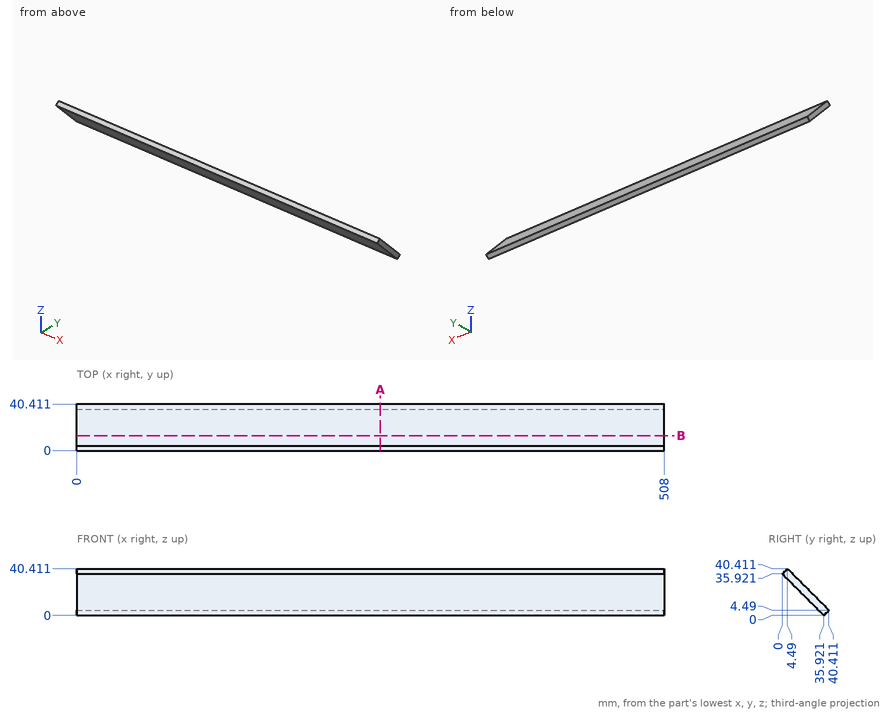
Verification items for this drawing (mm, ordinates from the low corner). Give positions to 0.01 mm unless a question says otherwise; leave off trailing zeros. Write each loop counter-clockwise with the first axis right and the second up, starting at its lowest first coordinate (ties: lowest second). Pieces come first, ordered by that corner, then holes.
1) Section check A-A, the plane x = 262.5. Record the boundary of the cut face in (y, z), and give its area (3 significant figures).
2) Material ranges on L1, parallel to Y at x = 208, z = 8.5; L2, parallel to Y at x = 54, z = 37; L3, parallel to Z at x = 226, y = 27, recorded low to high.
3) Gauge pin test, flat ends, axial feed: pin 1 (1 mm diameter, centred on x = 182.5, z = 27.5, fed in from +Y); pin 2 (1 mm diameter, centred on x = 241.5, y = 27.5, fed in from -Z); pin 3 (10 mm diameter, centred on x = 329, z = 29.5, fed in from -Y). Record the tip position at first contact, or that the pin passes through.
4) Section check B-B, the plane y = 13. Record the boundary of the cut face in (x, z), and give its area (3 significant figures).
Computed:
1. outline: (0, 35.92) - (35.92, 0) - (40.41, 4.49) - (4.49, 40.41) - close
1. area: 323 mm2
2. L1: y = 27.42 to 36.4
2. L2: y = 1.08 to 7.9
2. L3: z = 8.92 to 17.9
3. pin 1: stops at y = 17.9
3. pin 2: stops at z = 7.92
3. pin 3: stops at y = 1.42
4. outline: (0, 22.92) - (508, 22.92) - (508, 31.9) - (0, 31.9) - close
4. area: 4,560 mm2
